```python
from build123d import *

# Parameters (mm, degrees)
SKETCH1_W             = 130
SKETCH1_H             = 100
BOSS_EXTRUDE1_DEPTH   = 10
SKETCH2_R             = 45.5
BOSS_EXTRUDE2_DEPTH   = 65
SKETCH3_R             = 41
CUT_EXTRUDE1_DEPTH    = 76
SKETCH4_R             = 42.5
CUT_EXTRUDE2_DEPTH    = 35
M8_TAPPED_HOLE1_D     = 6.8
M8_TAPPED_HOLE1_DEPTH = 17.707073895
M8_TAPPED_HOLE1_TIP   = 2.042926105


with BuildPart() as part:
    # Sketch1 → Boss-Extrude1 (new body)
    with BuildSketch(Plane(origin=(0, 0, 0), x_dir=(1, 0, 0), z_dir=(0, 1, 0))):
        Rectangle(SKETCH1_W, SKETCH1_H)
    extrude(amount=BOSS_EXTRUDE1_DEPTH)

    # Sketch2 → Boss-Extrude2 (add)
    with BuildSketch(Plane(origin=(0, 10, 0), x_dir=(1, 0, 0), z_dir=(0, 1, 0))):
        Circle(SKETCH2_R)
    extrude(amount=BOSS_EXTRUDE2_DEPTH)

    # Sketch3 → Cut-Extrude1 (cut, through all)
    with BuildSketch(Plane(origin=(0, 75, 0), x_dir=(1, 0, 0), z_dir=(0, 1, 0))):
        Circle(SKETCH3_R)
    extrude(amount=-CUT_EXTRUDE1_DEPTH, mode=Mode.SUBTRACT)

    # Sketch4 → Cut-Extrude2 (cut)
    with BuildSketch(Plane.XZ):
        Circle(SKETCH4_R)
    extrude(amount=-CUT_EXTRUDE2_DEPTH, mode=Mode.SUBTRACT)

    # M8 Tapped Hole1
    with Locations(Plane(origin=(0, 10, 0), x_dir=(1, 0, 0), z_dir=(0, 1, 0))):
        with Locations((-50, 23.25), (-50, -23.25), (50, -23.25), (50, 23.25)):
            Hole(M8_TAPPED_HOLE1_D / 2, depth=M8_TAPPED_HOLE1_DEPTH)
            with Locations((0, 0, -(M8_TAPPED_HOLE1_DEPTH + M8_TAPPED_HOLE1_TIP / 2))):  # 118° drill point
                Cone(0, M8_TAPPED_HOLE1_D / 2, M8_TAPPED_HOLE1_TIP, mode=Mode.SUBTRACT)


solid = part.part
```
Geometry: final body of the model. Coordinates: model frame, mm. A direction names the side the tool comes from. Coordinates: 2 decimals unless noted, no trailing zeros. Order: outer loops, then holes, each group sorted by start corner. A loop starts at its lowest first (then second) coordinate and runs counter-clockwise, first axis right, second up. Notation, with made-up numbers: M 57,81 L 106,81 A24 cw 106,118 Z; hole C -27,4 d6. An arc over 180 degrees is marked long. Answer in a Markdown table with one row per item. Add a question column.
Q1. Section query D-D on x = -50. Return the cut outline in (y, z), and give its area (3 significant figures).
Q2. Line query: L1, parallel to Z at x = -50, y = 8; L2, parallel to X at y = 60, z = 0; L3, parallel to X at y = 8, z = 23.25. Output: solid intervals per line, ascending.
Q3. Contact query for flat-ended pins moving along their axis: P1, Ø3, axis at y = 41.5, z = -6, coming from the -X side; P2, Ø10, axis at y = 57, z = -20.5, coming from the +X side; P3, Ø2, axis at x = 34, y = 30.5, coming from the -Z side. Output: stop coordinate, or through.
Q4. Mould query, pull axis X, two halves, no side actions, for faces 1 (the flat face through (-1, 5, 50)), 2 (the cylindrical face through (-9, 55, 40)), 3 (the cylindrical face through (-36.107, 42.045, 27.686)), 4 (the cylindrical face through (-53.14, 4.93, -21.95)). Classes: released by +X, released by -X, zero draft, split by the parting line, or undercut.
Q5. Section query A-A on x = 0. Return the cut outline in (y, z), and give its area (3 significant figures).
Q6. Section query C-C on z = 11.5. Return the cut outline in (x, y).
Q7. Reachability of faces 5 (the cylindrical face through (-33.727, 17.255, -25.861)), 6 (the cylindrical face through (46.86, 4.93, -21.95)), 7 (the flat face through (-44.2, 10, -11.8)) from +Z, -Z, +X, -X, +Y, -Y: full face, straight path, thin tool, end or side. Return the list, or none.
Q8. Section query B-B on y = 6. Return the cut outline in (x, z), and give its area (3 significant figures).
Completed:
| question | item | result |
|---|---|---|
| 1 | outline | M 0,-50 L 10,-50 L 10,-26.65 L 0,-26.65 Z; M 0,-19.85 L 10,-19.85 L 10,19.85 L 0,19.85 Z; M 0,26.65 L 10,26.65 L 10,50 L 0,50 Z |
| 1 | area | 864 mm2 |
| 2 | L1 | z = -50 to -26.65, -19.85 to 19.85, 26.65 to 50 |
| 2 | L2 | x = -45.5 to -41, 41 to 45.5 |
| 2 | L3 | x = -65 to -53.4, -46.6 to -35.58, 35.58 to 46.6, 53.4 to 65 |
| 3 | P1 | stops at x = -45.28 |
| 3 | P2 | stops at x = 42.78 |
| 3 | P3 | stops at z = -31.32 |
| 4 | face 1 | zero draft |
| 4 | face 2 | undercut |
| 4 | face 3 | split by the parting line |
| 4 | face 4 | undercut |
| 5 | outline | M 0,-50 L 10,-50 L 10,-45.5 L 75,-45.5 L 75,-41 L 35,-41 L 35,-42.5 L 0,-42.5 Z; M 0,42.5 L 35,42.5 L 35,41 L 75,41 L 75,45.5 L 10,45.5 L 10,50 L 0,50 Z |
| 5 | area | 660 mm2 |
| 6 | outline | M -65,0 L -40.91,0 L -40.91,35 L -39.35,35 L -39.35,75 L -44.02,75 L -44.02,10 L -65,10 Z; M 39.35,35 L 40.91,35 L 40.91,0 L 65,0 L 65,10 L 44.02,10 L 44.02,75 L 39.35,75 Z |
| 7 | face 5 | -Y |
| 7 | face 6 | +Y, -Y |
| 7 | face 7 | +Y |
| 8 | outline | M -65,-50 L 65,-50 L 65,50 L -65,50 Z; hole C -50,-23.25 d6.8; hole C -50,23.25 d6.8; hole C 0,0 d85; hole C 50,-23.25 d6.8; hole C 50,23.25 d6.8 |
| 8 | area | 7,180 mm2 |
